The model under review builds one solid part; all positions refer to its coordinate system, in mm. A direction names the side the tool comes from. Coordinates: 2 decimals unless noted, no trailing zeros. Loops run counter-clockwise (first coordinate to the right, second up) from the corner with the lowest first, then second, coordinate; pieces in that order, holes last. Notation, with made-up numbers: (88, 56.25) - (104, 56.25) arc R28 ccw to (104, 91.25) - close; hole circle Ø4 at (67, 86). An arc over 180 degrees is marked (long way). Answer in a Markdown table with one row per item. Add a question column.
(1) We need section D-D on z = 0.85. Write out the cut boundary in (x, y).
(2) We need section A-A on x = 4.5. Write out the cut boundary in (y, z).
(3) For line 1 along Y through (x, z) = (4.5, 3.4); line 2 along Y through (x, z) = (4.5, 0.85); line 3 along X through (y, z) = (-25, 1.4), list the stretches that pass through material, from the lowest coordinate up.
(4) Mouldability with a two-part tool opening along Y and no side actions: class faces 1 (the flat face through (12, -20, 2)), 2 (the cylindrical face through (5.414, -23.567, 0.887)), 3 (the flat face through (6, 0, 2)) as +Y half, -Y half, draft (parallel to the pull), parting line (faces both ways), or undercut.
(5) Machinability: for faces 4 (the flat face through (7, -20, 4.8)), 5 (the cylindrical face through (4.149, -22.323, 3.279)), which of the approach directions +Z, -Z, +X, -X, +Y, -Y give a long, thin tool a straight path to every point of the face, cutting with its end or side? Answer none if there is none.
(6) We need section C-C on z = 3.6. Write out the cut boundary in (x, y), plus the area to 3 significant figures.
(7) For P1, Ø2, axis at y = -26, z = 2, coming from the -X side; P2, Ø1.6, axis at x = 6, y = -26, coming from the +Z side, all flat-tipped, find the tip position at first contact; note any pin that passes through.
(8) We need section B-B on y = -15. Write out the cut boundary in (x, z).
from build123d import *

# Parameters (mm, degrees)
CYLINDER1020_R     = 2.7
CYLINDER1020_DEPTH = 10
CYLINDER1018_R     = 1.7
CYLINDER1018_DEPTH = 10
PAD020_DEPTH       = 40


with BuildPart() as cylinder1015:
    # Cylinder1020 → Cylinder1020 (new body)
    with BuildSketch(Plane.XY.offset(10)):
        Circle(CYLINDER1020_R)
    extrude(amount=CYLINDER1020_DEPTH)


with BuildPart() as m3bolthead:
    # Cylinder1018 → Cylinder1018 (new body)
    with BuildSketch(Plane.XY):
        Circle(CYLINDER1018_R)
    extrude(amount=CYLINDER1018_DEPTH)

    # Fusion024: union Cylinder1015
    add(cylinder1015.part)


with BuildPart() as clone_of_m3bolthead002:
    # Clone034 base: copy of M3BoltHead
    add(m3bolthead.part)


with BuildPart() as clone_of_m3bolthead002_1:
    # Clone034 placement: moved
    add(clone_of_m3bolthead002.part.moved(Location((4.5, -15, -8.2))))


with BuildPart() as fusion041:
    # Clone033 base: copy of M3BoltHead
    add(m3bolthead.part)


with BuildPart() as fusion041_1:
    # Clone033 placement: moved
    add(fusion041.part.moved(Location((4.5, -25, -8.2))))

    # Fusion041: union Clone of M3BoltHead002
    add(clone_of_m3bolthead002_1.part)


with BuildPart() as obj1:
    # Sketch021 → Pad020 (new body)
    with BuildSketch(Plane.XZ):
        Polygon((0, 0), (0, 4.8), (14.8, 4.8), (10, 0), align=None)
    extrude(amount=PAD020_DEPTH)

    # Cut050: cut Fusion041
    add(fusion041_1.part, mode=Mode.SUBTRACT)


solid = obj1.part
Outcome:
| question | item | result |
|---|---|---|
| 1 | outline | (0, -40) - (10.85, -40) - (10.85, 0) - (0, 0) - close; hole circle Ø3.4 at (4.5, -25); hole circle Ø3.4 at (4.5, -15) |
| 2 | outline | (-40, 0) - (-26.7, 0) - (-26.7, 1.8) - (-27.7, 1.8) - (-27.7, 4.8) - (-40, 4.8) - close; (-23.3, 0) - (-16.7, 0) - (-16.7, 1.8) - (-17.7, 1.8) - (-17.7, 4.8) - (-22.3, 4.8) - (-22.3, 1.8) - (-23.3, 1.8) - close; (-13.3, 0) - (0, 0) - (0, 4.8) - (-12.3, 4.8) - (-12.3, 1.8) - (-13.3, 1.8) - close |
| 3 | line 1 | -40 to -27.7, -22.3 to -17.7, -12.3 to 0 |
| 3 | line 2 | -40 to -26.7, -23.3 to -16.7, -13.3 to 0 |
| 3 | line 3 | 0 to 2.8, 6.2 to 11.4 |
| 4 | face 1 | draft |
| 4 | face 2 | undercut |
| 4 | face 3 | +Y half |
| 5 | face 4 | +Z, +X, -X, +Y, -Y |
| 5 | face 5 | +Z |
| 6 | outline | (0, -40) - (13.6, -40) - (13.6, 0) - (0, 0) - close; hole circle Ø5.4 at (4.5, -25); hole circle Ø5.4 at (4.5, -15) |
| 6 | area | 498 mm² |
| 7 | P1 | x = 0 |
| 7 | P2 | z = 1.8 |
| 8 | outline | (0, 0) - (2.8, 0) - (2.8, 1.8) - (1.8, 1.8) - (1.8, 4.8) - (0, 4.8) - close; (6.2, 0) - (10, 0) - (14.8, 4.8) - (7.2, 4.8) - (7.2, 1.8) - (6.2, 1.8) - close |
